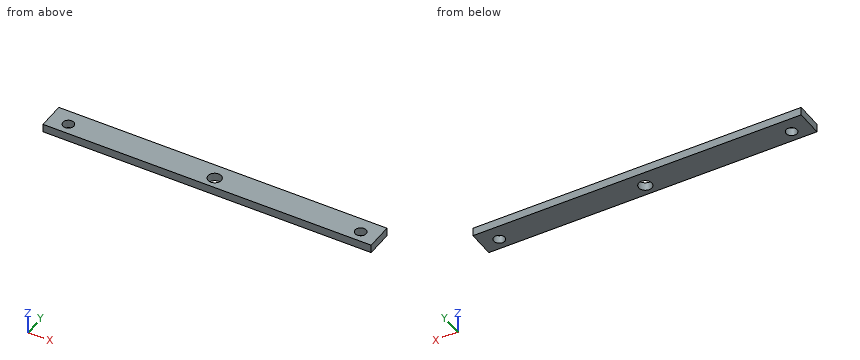
```python
from build123d import *

# Parameters (mm, degrees)
SKETCH1_W            = 158.980651351
SKETCH1_H            = 13.078234564
BOSS_EXTRUDE1_DEPTH  = 4
M5_CLEARANCE_HOLE1_D = 5.3
M6_CLEARANCE_HOLE2_D = 6.4


with BuildPart() as part:
    # Sketch1 → Boss-Extrude1 (new body)
    with BuildSketch(Plane.XY):
        with Locations((16.171323843, -296.4446159)):
            Rectangle(SKETCH1_W, SKETCH1_H)
    extrude(amount=BOSS_EXTRUDE1_DEPTH)

    # M5 Clearance Hole1 (through all)
    with Locations(Plane.XY.offset(4)):
        with Locations((87.370998167, -297.523461342), (-54.209001833, -297.523461342)):
            Hole(M5_CLEARANCE_HOLE1_D / 2)

    # M6 Clearance Hole2 (through all)
    with Locations(Plane.XY.offset(4)):
        with Locations((16.634702444, -297.523461342)):
            Hole(M6_CLEARANCE_HOLE2_D / 2)


solid = part.part
```
CAD build for the part. Positions are in the model's coordinates, mm. Round coordinates to 2 decimals unless told otherwise and drop trailing zeros. Write each loop counter-clockwise with the first axis right and the second up, starting at its lowest first coordinate (ties: lowest second). Pieces come first, ordered by that corner, then holes. Notation, with made-up numbers: M 7,-23.75 L 19,-23.75 A20 cw 19,-12.75 Z; hole C 59.5,-35 d2. An arc over 180 degrees is marked long. One line per question, with ' | ' between items.
1. Probe L1, parallel to X at y = -296.25, z = 3; L2, parallel to X at y = -296, z = 1.45; L3, parallel to Y at x = 87, z = 2.7. List the from-to ranges inside material, lowest first. Write a range as from..to.
Working result:
L1: -63.32..-56.53, -51.89..13.7, 19.57..85.05, 89.69..95.66 | L2: -63.32..-56.38, -52.04..13.82, 19.45..85.2, 89.54..95.66 | L3: -302.98..-300.15, -294.9..-289.91
2. Pin check, flat tip, straight feed: pin 1 Ø3 at (x, y) = (87.37, -297.52) entering from -Z. Stop position of the tip, or through.
Working result:
pin 1: through
3. Cut at A-A on z = 1.65. Write the cut outline in (x, y), and give its area (3 significant figures).
Working result:
outline: M -63.32,-302.98 L 95.66,-302.98 L 95.66,-289.91 L -63.32,-289.91 Z; hole C -54.21,-297.52 d5.3; hole C 16.63,-297.52 d6.4; hole C 87.37,-297.52 d5.3 | area: 2,000 mm2
